```python
from build123d import *
from build123d.topology import SkipClean

# Parameters (mm, degrees)
BOSS_EXTRUDE1_DEPTH      = 5
BOSS_EXTRUDE2_START      = -5
SKETCH3_R                = 7.5
BOSS_EXTRUDE2_DEPTH      = 11
SKETCH7_R                = 2.5
BOSS_EXTRUDE7_DEPTH      = 3
SKETCH8_R                = 4.5
BOSS_EXTRUDE8_DEPTH      = 3
BOSS_EXTRUDE9_DEPTH      = 8
BOSS_EXTRUDE9_DEPTH_BACK = 2
BOSS_EXTRUDE9_START      = 65
SKETCH9_R                = 2.5
SKETCH4_R                = 4.5
CUT_EXTRUDE1_DEPTH       = 117.364534493


with BuildPart() as part:
    # Sketch1 → Boss-Extrude1 (new body)
    with BuildSketch(Plane.XY):
        with BuildLine():
            Line((-5, 95), (-5, 0))
            Line((-5, 0), (0, 0))
            Line((0, 0), (0, 99.161508865))
            ThreePointArc((0, 99.161508865), (-4.5, 103.661508865), (0, 108.161508865))
            Line((0, 108.161508865), (0, 113.662595596))
            ThreePointArc((0, 113.662595596), (-9.660389154, 106.249677564), (-5, 95))
        make_face()
    boss_extrude1 = extrude(amount=BOSS_EXTRUDE1_DEPTH)

    # Sketch3 → Boss-Extrude2 (add)
    with BuildSketch(Plane.ZY.offset(5).offset(BOSS_EXTRUDE2_START)):
        with Locations(Location((0, 5.43173798, 0), (0, 0, 270))):
            Circle(SKETCH3_R)
    boss_extrude2 = extrude(amount=BOSS_EXTRUDE2_DEPTH)

    # Sketch7 → Boss-Extrude7 (add)
    with BuildSketch(Plane(origin=(0, 0, 0), x_dir=(-1, 0, 0), z_dir=(0, 0, -1))):
        with Locations(Location((0, 46.751317941, 0), (0, 0, 270))):
            Circle(SKETCH7_R)
    extrude(amount=BOSS_EXTRUDE7_DEPTH)

    # Sketch8 → Boss-Extrude8 (add)
    with BuildSketch(Plane(origin=(0, 0, -3), x_dir=(-1, 0, 0), z_dir=(0, 0, -1))):
        with Locations((0, 46.751317941)):
            Circle(SKETCH8_R)
    extrude(amount=BOSS_EXTRUDE8_DEPTH)

    # Sketch9 → Boss-Extrude9 (add, two sides: drawn at the far end of the back side and taken through both)
    with BuildSketch(Plane(origin=(0, 0, 0), x_dir=(1, 0, 0), z_dir=(0, 1, 0)).offset(BOSS_EXTRUDE9_START - BOSS_EXTRUDE9_DEPTH_BACK)):
        with BuildLine():
            Line((-3.3634301, -8.3634301), (-3.3634301, -5))
            Line((-3.3634301, -5), (3.3634301, -5))
            Line((3.3634301, -5), (3.3634301, -8.3634301))
            ThreePointArc((3.3634301, -8.3634301), (0, -11.726860201), (-3.3634301, -8.3634301))
        make_face()
        with Locations(Location((0, -8.3634301, 0), (0, 0, 270))):
            Circle(SKETCH9_R, mode=Mode.SUBTRACT)
    extrude(amount=BOSS_EXTRUDE9_DEPTH + BOSS_EXTRUDE9_DEPTH_BACK)

    # Mirror1: Boss-Extrude1, Boss-Extrude2 across plane
    with SkipClean():  # the faces are left unmerged after this step: merging them gives an invalid solid
        add(boss_extrude1.mirror(Plane(origin=(0, 0, 5), x_dir=(0, 0, 1), z_dir=(-1, 0, 0))))
        add(boss_extrude2.mirror(Plane(origin=(0, 0, 5), x_dir=(0, 0, 1), z_dir=(-1, 0, 0))))

    # Sketch4 → Cut-Extrude1 (cut, through all)
    with SkipClean():  # the faces are left unmerged after this step: merging them gives an invalid solid
        with BuildSketch(Plane.ZY.offset(11)):
            with Locations(Location((0, 5.43173798, 0), (0, 0, 270))):
                Circle(SKETCH4_R)
        extrude(amount=-CUT_EXTRUDE1_DEPTH, mode=Mode.SUBTRACT)


solid = part.part
```
CAD build for the part. Positions are in the model's coordinates, mm. A direction names the side the tool comes from. Round coordinates to 2 decimals unless told otherwise and drop trailing zeros. Write each loop counter-clockwise with the first axis right and the second up, starting at its lowest first coordinate (ties: lowest second). Pieces come first, ordered by that corner, then holes. Notation, with made-up numbers: (89, 24.5) - (119, 24.5) arc R37 ccw to (119, 60.5) - close; hole circle Ø11 at (51.5, -28.75). An arc over 180 degrees is marked (long way). Write item = value, one per line. Start each with the question number.
Q1. Band-saw the part on A-A (x = 6). Give the cut face in (y, z), then the cut area to 3 significant figures.
Q2. Drop flat-ended pins along their axis: pin 1 (5 mm diameter, centred on y = 82, z = -4.5, fed in from -X); pin 2 (4.5 mm diameter, centred on x = -2, y = 44.5, fed in from -Z); pin 3 (7 mm diameter, centred on x = -2, y = 45.5, fed in from +Z); pin 4 (2.5 mm diameter, centred on y = 70.5, z = 7.5, fed in from +X). Give the stop position or say it passes through.
Q3. Band-saw the part on C-C (y = 71.5). Give the cut face in (x, z), then the cut area to 3 significant figures.
Q4. Which spindle directions (+Z, -Z, +X, -X, +Y, -Y) get a long thin tool onto all of the face, cutting with end or side? Do faces 5 (the cylindrical face through (0.958, 44.442, -1.479)), 6 (the cylindrical face through (0.586, 51.213, -4.479)), 7 (the flat face through (0, 47, -6)). Say none if no direction does.
Q5. Probe L1, parallel to Z at x = 2.25, y = 5; L2, parallel to X at y = 45, z = 3.5; L3, parallel to Z at x = 1.25, y = 78. List the from-to ranges inside material, lowest first. Write a range as from..to.
Q6. Mould opens along Z. For faces 1 (the flat face through (-2, 45, -3)), 2 (the cylindrical face through (0.074, 67.93, 11.726)), 3 (the cylindrical face through (0.11, 67.93, 5.866)), 4 (the flat face through (-1.4, 73, 6.1)) say: pulls with the +Z half, pulls with the -Z half, needs draft (parallel to the pull), parting line crosses it, or undercut.
Q7. Band-saw the part on B-B (z = 1). Give the cut face in (x, y), then the cut area to 3 significant figures.
Q8. Band-saw the part on D-D (x = -9). Give the cut face in (y, z), then the cut area to 3 significant figures.
Answers below:
q1.outline = circle Ø15 at (5.43, 0); (95.66, 0) - (111.66, 0) - (111.66, 5) - (95.66, 5) - close; hole circle Ø9 at (5.43, 0)
q1.area = 193 mm2
q2.pin_1 = through
q2.pin_2 = -6
q2.pin_3 = 5
q2.pin_4 = 3.36
q3.outline = (-5, 0) - (5, 0) - (5, 5) - (3.36, 5) - (3.36, 8.36) arc R3.36 ccw to (-3.36, 8.36) - (-3.36, 5) - (-5, 5) - close; hole circle Ø5 at (0, 8.36)
q3.area = 70.8 mm2
q4.face_5 = none
q4.face_6 = -Z
q4.face_7 = -Z, +X, -X, +Y
q5.L1 = -7.49..-4.48, 4.48..7.49
q5.L2 = -5..5
q5.L3 = 0..5
q6.face_1 = undercut
q6.face_2 = pulls with the +Z half
q6.face_3 = undercut
q6.face_4 = needs draft
q7.outline = (-11, -2) - (11, -2) - (11, 1.04) - (-11, 1.04) - close; (-11, 9.82) - (11, 9.82) - (11, 12.86) - (5, 12.86) - (5, 95) arc R10 ccw (long way) to (-5, 95) - (-5, 12.86) - (-11, 12.86) - close; hole circle Ø9 at (0, 103.66)
q7.area = 1,200 mm2
q8.outline = circle Ø15 at (5.43, 0); (99.3, 0) - (108.02, 0) - (108.02, 5) - (99.3, 5) - close; hole circle Ø9 at (5.43, 0)
q8.area = 157 mm2
